Could you check a few things on this model? Use its own coordinates, in mm. Face numbers are marked on the shaded views. Round coordinates to 2 decimals unless told otherwise and drop trailing zeros. Write each loop counter-clockwise with the first axis right and the second up, starting at its lowest first coordinate (ties: lowest second). Pieces come first, ordered by that corner, then holes. Notation, with made-up numbers: (27, -26.5) -> (53, -26.5) arc R10 cw to (53, -13.5) -> close; hole circle Ø1 at (40, 77). An arc over 180 degrees is marked (long way). One line per question, with ' | ' between items. Start each with the question number.
1. Imagine slicing it at D-D, the plane z = 15. List the corners of the cut face in (x, y) for me, and give its area (3 significant figures).
2. Imagine slicing it at A-A, the plane x = 0. List the corners of the cut face in (y, z) for me, and give its area (3 significant figures).
3. If I drill on line 1 along X through (y, z) = (8, 91); line 2 along Y through (x, z) = (0, 22); line 3 along X through (y, z) = (-10, 17), over which ranges is the centre line in solid material (lowest first)? Write a range as [from, to].
4. For pin 1 Ø15.5 at (y, z) = (-14, 57.5) entering from +X; pin 2 Ø3 at (y, z) = (-17.5, 85) entering from -X; pin 3 Ø9.5 at (x, z) = (-11, 30.5) entering from -Y; pin 4 Ø5.5 at (x, y) = (0, 0) entering from -Z, each with a flat end and sliding along its axis, tell me the tip position at first contact or that it passes through.
5. Thinking about a two-plate mould opening in X: for the marked faces 1 and 2, which applies, released by +X, released by -X, zero draft, split by the parting line, or undercut?
6. Imagine slicing it at C-C, the plane x = -11. List the corners of the cut face in (y, z) for me.
from build123d import *

# Parameters (mm, degrees)
F0_R     = 26
F0_R_2   = 4.5
F1_DEPTH = 100


with BuildPart() as f1:
    # F0 (on Top) → F1 (new body)
    with BuildSketch(Plane.XY):
        Circle(F0_R)
        with BuildLine():
            ThreePointArc((24.454039, 1.5), (24.488507, 0.750352), (24.5, 0))
            ThreePointArc((24.5, 0), (24.488507, -0.750352), (24.454039, -1.5))
            ThreePointArc((24.454039, -1.5), (17.324116, -17.324116), (1.5, -24.454039))
            ThreePointArc((1.5, -24.454039), (0.750352, -24.488507), (0, -24.5))
            ThreePointArc((0, -24.5), (-0.750352, -24.488507), (-1.5, -24.454039))
            ThreePointArc((-1.5, -24.454039), (-17.324116, -17.324116), (-24.454039, -1.5))
            ThreePointArc((-24.454039, -1.5), (-24.488507, -0.750352), (-24.5, 0))
            ThreePointArc((-24.5, 0), (-24.488507, 0.750352), (-24.454039, 1.5))
            ThreePointArc((-24.454039, 1.5), (-17.324116, 17.324116), (-1.5, 24.454039))
            ThreePointArc((-1.5, 24.454039), (-0.750352, 24.488507), (0, 24.5))
            ThreePointArc((0, 24.5), (0.750352, 24.488507), (1.5, 24.454039))
            ThreePointArc((1.5, 24.454039), (17.324116, 17.324116), (24.454039, 1.5))
        make_face(mode=Mode.SUBTRACT)
        with BuildLine():
            Line((0, 5.5), (0, 24.5))
            ThreePointArc((0, 24.5), (-0.750352, 24.488507), (-1.5, 24.454039))
            Line((-1.5, 24.454039), (-1.5, 5.291503))
            ThreePointArc((-1.5, 5.291503), (-0.757211, 5.447626), (0, 5.5))
        make_face()
        with BuildLine():
            Line((1.5, 5.291503), (1.5, 24.454039))
            ThreePointArc((1.5, 24.454039), (0.750352, 24.488507), (0, 24.5))
            Line((0, 24.5), (0, 5.5))
            ThreePointArc((0, 5.5), (0.757211, 5.447626), (1.5, 5.291503))
        make_face()
        with BuildLine():
            ThreePointArc((5.291503, -1.5), (5.447626, -0.757211), (5.5, 0))
            ThreePointArc((5.5, 0), (5.447626, 0.757211), (5.291503, 1.5))
            ThreePointArc((5.291503, 1.5), (3.889087, 3.889087), (1.5, 5.291503))
            ThreePointArc((1.5, 5.291503), (0.757211, 5.447626), (0, 5.5))
            ThreePointArc((0, 5.5), (-0.757211, 5.447626), (-1.5, 5.291503))
            ThreePointArc((-1.5, 5.291503), (-3.889087, 3.889087), (-5.291503, 1.5))
            ThreePointArc((-5.291503, 1.5), (-5.447626, 0.757211), (-5.5, 0))
            ThreePointArc((-5.5, 0), (-5.447626, -0.757211), (-5.291503, -1.5))
            ThreePointArc((-5.291503, -1.5), (-3.889087, -3.889087), (-1.5, -5.291503))
            ThreePointArc((-1.5, -5.291503), (-0.757211, -5.447626), (0, -5.5))
            ThreePointArc((0, -5.5), (0.757211, -5.447626), (1.5, -5.291503))
            ThreePointArc((1.5, -5.291503), (3.889087, -3.889087), (5.291503, -1.5))
        make_face()
        Circle(F0_R_2, mode=Mode.SUBTRACT)
        with BuildLine():
            Line((5.5, 0), (24.5, 0))
            ThreePointArc((24.5, 0), (24.488507, 0.750352), (24.454039, 1.5))
            Line((24.454039, 1.5), (5.291503, 1.5))
            ThreePointArc((5.291503, 1.5), (5.447626, 0.757211), (5.5, 0))
        make_face()
        with BuildLine():
            ThreePointArc((24.454039, -1.5), (24.488507, -0.750352), (24.5, 0))
            Line((24.5, 0), (5.5, 0))
            ThreePointArc((5.5, 0), (5.447626, -0.757211), (5.291503, -1.5))
            Line((5.291503, -1.5), (24.454039, -1.5))
        make_face()
        with BuildLine():
            ThreePointArc((-1.5, -24.454039), (-0.750352, -24.488507), (0, -24.5))
            Line((0, -24.5), (0, -5.5))
            ThreePointArc((0, -5.5), (-0.757211, -5.447626), (-1.5, -5.291503))
            Line((-1.5, -5.291503), (-1.5, -24.454039))
        make_face()
        with BuildLine():
            Line((-5.291503, 1.5), (-24.454039, 1.5))
            ThreePointArc((-24.454039, 1.5), (-24.488507, 0.750352), (-24.5, 0))
            Line((-24.5, 0), (-5.5, 0))
            ThreePointArc((-5.5, 0), (-5.447626, 0.757211), (-5.291503, 1.5))
        make_face()
        with BuildLine():
            ThreePointArc((-24.5, 0), (-24.488507, -0.750352), (-24.454039, -1.5))
            Line((-24.454039, -1.5), (-5.291503, -1.5))
            ThreePointArc((-5.291503, -1.5), (-5.447626, -0.757211), (-5.5, 0))
            Line((-5.5, 0), (-24.5, 0))
        make_face()
        with BuildLine():
            ThreePointArc((0, -24.5), (0.750352, -24.488507), (1.5, -24.454039))
            Line((1.5, -24.454039), (1.5, -5.291503))
            ThreePointArc((1.5, -5.291503), (0.757211, -5.447626), (0, -5.5))
            Line((0, -5.5), (0, -24.5))
        make_face()
    extrude(amount=F1_DEPTH)


solid = f1.part
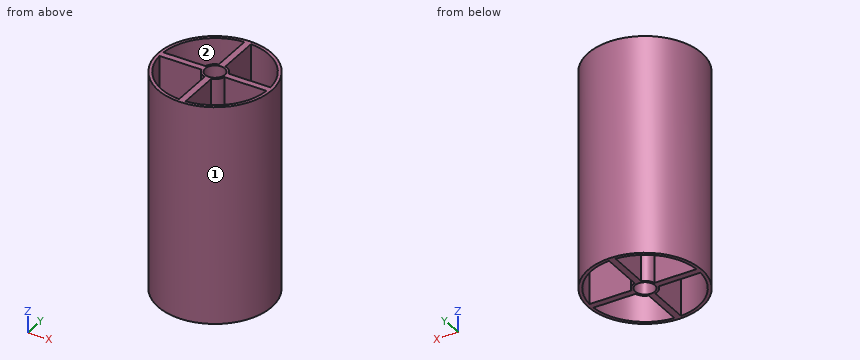
Geometry results:
1) outline: circle Ø52 at (0, 0); hole (-24.45, -1.5) arc R24.5 ccw to (-1.5, -24.45) -> (-1.5, -5.29) arc R5.5 cw to (-5.29, -1.5) -> close; hole (-24.45, 1.5) -> (-5.29, 1.5) arc R5.5 cw to (-1.5, 5.29) -> (-1.5, 24.45) arc R24.5 ccw to start; hole circle Ø9 at (0, 0); hole (1.5, -24.45) arc R24.5 ccw to (24.45, -1.5) -> (5.29, -1.5) arc R5.5 cw to (1.5, -5.29) -> close; hole (1.5, 5.29) arc R5.5 cw to (5.29, 1.5) -> (24.45, 1.5) arc R24.5 ccw to (1.5, 24.45) -> close | area: 498 mm2
2) outline: (-26, 0) -> (-4.5, 0) -> (-4.5, 100) -> (-26, 100) -> close; (4.5, 0) -> (26, 0) -> (26, 100) -> (4.5, 100) -> close | area: 4,300 mm2
3) line 1: x = [-24.74, -23.16], [-1.5, 1.5], [23.16, 24.74] | line 2: y = [-26, -4.5], [4.5, 26] | line 3: x = [-24, -22.37], [-1.5, 1.5], [22.37, 24]
4) pin 1: stops at x = 25.24 | pin 2: stops at x = -20.49 | pin 3: stops at y = -25.24 | pin 4: passes through
5) face 1: split by the parting line | face 2: undercut
6) outline: (-23.56, 0) -> (-21.89, 0) -> (-21.89, 100) -> (-23.56, 100) -> close; (-1.5, 0) -> (1.5, 0) -> (1.5, 100) -> (-1.5, 100) -> close; (21.89, 0) -> (23.56, 0) -> (23.56, 100) -> (21.89, 100) -> close
